```python
from build123d import *

# Parameters (mm, degrees)
FILLET2_R  = 1.5
SKETCH2_W  = 9.5
SKETCH2_H  = 1.2
SLOT_DEPTH = 1.2


with BuildPart() as part:
    # BodySke → Base-Revolve (revolve)
    with BuildSketch(Plane.XY, mode=Mode.PRIVATE) as base_revolve_sk:
        Polygon((3, 2.5), (3, 4.75), (0, 4.487534009), (0, 0), (13, 0), (13, 2.5), align=None)
    revolve(base_revolve_sk.sketch.rotate(Axis((-25.4, 0, 0), (1, 0, 0)), 90), axis=Axis((-25.4, 0, 0), (1, 0, 0)))  # turned: the seam where the file's is

    # Fillet2
    fillet2_edges = [part.edges().sort_by_distance(p)[0] for p in [
        (0, 0, -4.487534009),
    ]]
    fillet(fillet2_edges, radius=FILLET2_R)

    # Sketch2 → Slot (cut)
    with BuildSketch(Plane(origin=(0, 0, 0), x_dir=(0, 0, -1), z_dir=(1, 0, 0))):
        Rectangle(SKETCH2_W, SKETCH2_H)
    extrude(amount=SLOT_DEPTH, mode=Mode.SUBTRACT)


solid = part.part
```
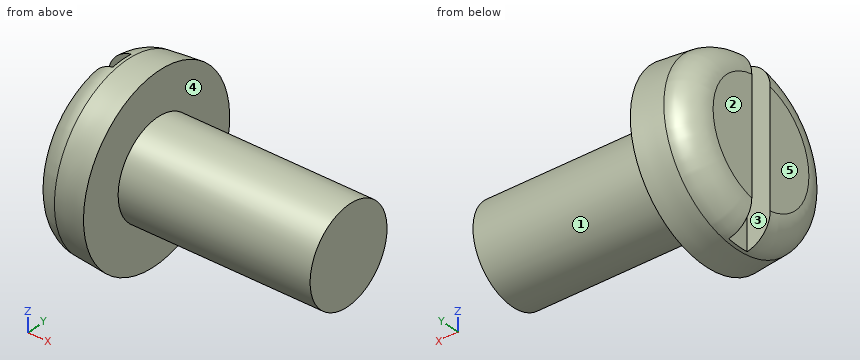
Part model, mm, in its own coordinate system. Face numbers are marked on the shaded views. A direction names the side the tool comes from. Coordinates: 2 decimals unless noted, no trailing zeros. Loops run counter-clockwise (first coordinate to the right, second up) from the corner with the lowest first, then second, coordinate; pieces in that order, holes last. Notation, with made-up numbers: (16, 46) - (56, 46) arc R23 cw to (56, 78) - close; hole circle Ø8 at (-25, 20.5). An arc over 180 degrees is marked (long way). Write item = value, one per line. Start each with the question number.
Item 1: Wall check: L1, parallel to X at y = 2.25, z = 2; L2, parallel to Y at x = 1, z = -0.5; L3, parallel to Y at x = 0.5, z = 0.75. Give the ranges that are in metal, low to high. Write a range as from..to.
Item 2: Cut at B-B, the plane z = 0. Give the cut face in (x, y), and give its area (3 significant figures).
Item 3: 3-axis set-ups, long thin cutter, end or side, ignore diameter. For the marked faces 4 and 5: which of +Z, -Z, +X, -X, +Y, -Y reach the whole face in a straight line?
Item 4: Cut at A-A, the plane y = 0. Give the cut face in (x, z), and give its area (3 significant figures).
Item 5: Cut at C-C, the plane x = 4.25. Give the cut face in (y, z), and give its area (3 significant figures).
Item 6: Cut at D-D, the plane x = 2.5. Give the cut face in (y, z).
Item 7: Flat gauge pins, fed straight in: pin 1 Ø1 at (x, z) = (11, 0) entering from -Y; pin 2 Ø1.3 at (x, z) = (0.5, 1.5) entering from +Y; pin 3 Ø1.3 at (x, z) = (0.5, 0.5) entering from -Y. Where does each tip first touch, or does it go through?
Item 8: Mould opens along Y. For the marked faces 1, 2 and 3 say: released by +Y, released by -Y, zero draft, split by the parting line, or undercut.
The answers:
q1.L1 = 0..3
q1.L2 = -4.5..-0.6, 0.6..4.5
q1.L3 = -4.16..-0.6, 0.6..4.16
q2.outline = (0, -3.11) arc R1.5 ccw to (1.37, -4.61) - (3, -4.75) - (3, -2.5) - (13, -2.5) - (13, 2.5) - (3, 2.5) - (3, 4.75) - (1.37, 4.61) arc R1.5 ccw to (0, 3.11) - (0, 0.6) - (1.2, 0.6) - (1.2, -0.6) - (0, -0.6) - close
q2.area = 75.5 mm2
q3.face_4 = +X
q3.face_5 = +Z, -Z, -X, +Y, -Y
q4.outline = (1.2, -4.58) arc R1.5 ccw to (1.37, -4.61) - (3, -4.75) - (3, -2.5) - (13, -2.5) - (13, 2.5) - (3, 2.5) - (3, 4.75) - (1.37, 4.61) arc R1.5 ccw to (1.2, 4.58) - close
q4.area = 66.8 mm2
q5.outline = circle Ø5 at (0, 0)
q5.area = 19.6 mm2
q6.outline = circle Ø9.41 at (0, 0)
q7.pin_1 = -2.5
q7.pin_2 = 4.4
q7.pin_3 = -4.55
q8.face_1 = split by the parting line
q8.face_2 = zero draft
q8.face_3 = undercut
